Source: three-view drawing plus pictorial views. Frame: mm from the lowest corner of the part. A direction names the side the tool comes from. Round coordinates to 2 decimals unless told otherwise and drop trailing zeros. Loops run counter-clockwise (first coordinate to the right, second up) from the corner with the lowest first, then second, coordinate; pieces in that order, holes last. Notation, with made-up numbers: M -28.75,20 L -16.75,20 A27 ccw -16.75,44 Z; hole C 56,6.5 d3. An arc over 180 degrees is marked long. Answer as a JSON object with one key per item and string values.
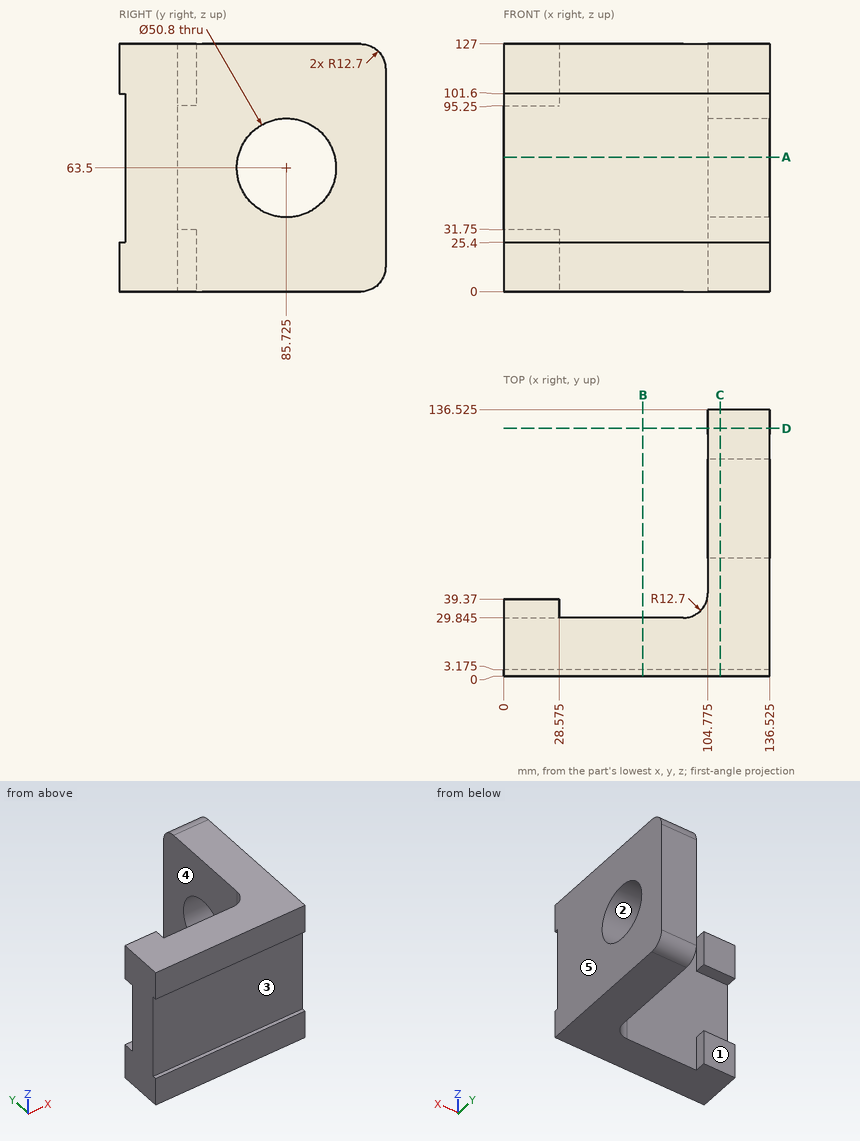
1) Set-up query: the marked faces 4 and 5. Return all of +Z, -Z, +X, -X, +Y, -Y with unobstructed straight access to the full face (end or side cutting, diameter ignored); none if empty.
Geometry results:
{"face 4": "+Z, -Z, -X, +Y", "face 5": "+Z, -Z, +X, +Y, -Y"}
2) Cut plane B-B on x = 71.5. Return the cut outline in (y, z) (3 decimals).
Geometry results:
{"outline": "M 0,0 L 29.845,0 L 29.845,127 L 0,127 L 0,101.6 L 3.175,101.6 L 3.175,25.4 L 0,25.4 Z"}
3) Cut plane A-A on z = 69. Return the cut outline in (x, y) (3 decimals).
Geometry results:
{"outline": "M 0,3.175 L 136.525,3.175 L 136.525,60.928 L 104.775,60.928 L 104.775,42.545 A12.7 cw 92.075,29.845 L 0,29.845 Z; M 104.775,110.522 L 136.525,110.522 L 136.525,136.525 L 104.775,136.525 Z"}
4) Cut plane C-C on x = 111. Return the cut outline in (y, z) (3 decimals).
Geometry results:
{"outline": "M 0,0 L 123.825,0 A12.7 ccw 136.525,12.7 L 136.525,114.3 A12.7 ccw 123.825,127 L 0,127 L 0,101.6 L 3.175,101.6 L 3.175,25.4 L 0,25.4 Z; hole C 85.725,63.5 d50.8"}
5) Pull-direction query (Y, two-part tool) for the marked faces 1, 2 and 3; classes: +Y half, -Y half, draft (parallel to the pull), parting line (faces both ways), or undercut.
Geometry results:
{"face 1": "+Y half", "face 2": "undercut", "face 3": "-Y half"}
6) Cut plane D-D on y = 127. Return the cut outline in (x, z) (3 decimals), and give its area (3 significant figures).
Geometry results:
{"outline": "M 104.775,0.403 L 136.525,0.403 L 136.525,126.597 L 104.775,126.597 Z", "area": "4,010 mm2"}
7) Line query: probe 1 along Y at (x, z) = (117, 63) (3 decimals); probe 2 along X at (y, z) = (63, 113) (3 decimals); probe 3 along Y at (x, z) = (76, 58.5) (3 decimals). Output: solid intervals per line, ascending.
Geometry results:
{"probe 1": "3.175 to 60.33, 111.12 to 136.525", "probe 2": "104.775 to 136.525", "probe 3": "3.175 to 29.845"}
8) First-contact query: pin 1 (12 mm diameter, centred on x = 71, z = 17, fed in from +Y) (3 decimals); pin 2 (5 mm diameter, centred on x = 9.5, y = 33, fed in from -Z); pin 3 (23 mm diameter, centred on x = 12.5, z = 15, fed in from +Y); pin 4 (3 mm diameter, centred on x = 44, z = 41.5, fed in from -Y) (3 decimals). Flat tips, straight axial feed; report the tip coordinate or a pass-through.
Geometry results:
{"pin 1": "y = 29.845", "pin 2": "z = 0", "pin 3": "y = 39.37", "pin 4": "y = 3.175"}
